Source: CAD feature listing. Evaluate the final solid. Frame: model axes, mm. Face numbers are marked on the shaded views. Give positions to 0.01 mm unless a question says otherwise; leave off trailing zeros. Order: outer loops, then holes, each group sorted by start corner. A loop starts at its lowest first (then second) coordinate and runs counter-clockwise, first axis right, second up. Notation, with made-up numbers: (45, 33) -> (78, 33) arc R16 cw to (78, 61) -> close; hole circle Ø8 at (36.25, 8). An arc over 180 degrees is marked (long way). Answer in a Markdown table with one row per item.
```python
from build123d import *

# Parameters (mm, degrees)
F0_R     = 11
F1_DEPTH = 7


with BuildPart() as f1:
    # F0 (on Top) → F1 (new body)
    with BuildSketch(Plane.XY):
        with BuildLine():
            ThreePointArc((14.1759402298, -3.0483960701), (14.4187574592, -1.5327861344), (14.5, 0))
            ThreePointArc((14.5, 0), (14.421984404, 1.5021204517), (14.188777124, 2.9880769278))
            add(Edge.make_bspline(
                [(14.0117061641, 3.7312317498), (14.0561894605, 3.4787953407), (14.1150221965, 3.2304441785), (14.188777124, 2.9880769278)],
                knots=[0.9498383363, 0.9498383363, 0.9498383363, 0.9498383363, 1, 1, 1, 1], degree=3))
            ThreePointArc((14.0117061641, 3.7312317498), (7.1105429941, 12.6368579295), (-4.0835358776, 13.9131137685))
            add(Edge.make_bspline(
                [(-4.0835358776, 13.9131137685), (-4.9864056262, 13.4237848609), (-5.8861011392, 13.0613615019), (-6.6725668518, 12.8734941492)],
                knots=[0.8398981571, 0.8398981571, 0.8398981571, 0.8398981571, 1, 1, 1, 1], degree=3))
            ThreePointArc((-6.6725668518, 12.8734941492), (-7.25, 12.5573683549), (-7.8124895427, 12.2153594767))
            add(Edge.make_bspline(
                [(-10.3373118209, 10.1680865613), (-9.3752684105, 10.9198780403), (-8.503153556, 11.689001034), (-7.8124895427, 12.2153594767)],
                knots=[0.8153153807, 0.8153153807, 0.8153153807, 0.8153153807, 1, 1, 1, 1], degree=3))
            ThreePointArc((-10.3373118209, 10.1680865613), (-14.5, 0), (-10.3373118209, -10.1680865613))
            add(Edge.make_bspline(
                [(-10.3373118209, -10.1680865613), (-9.3752684105, -10.9198780403), (-8.503153556, -11.689001034), (-7.8124895427, -12.2153594767)],
                knots=[0.8153153807, 0.8153153807, 0.8153153807, 0.8153153807, 1, 1, 1, 1], degree=3))
            ThreePointArc((-7.8124895427, -12.2153594767), (-6.1812855522, -13.1164670899), (-4.4479816774, -13.8009223966))
            add(Edge.make_bspline(
                [(-3.7286645674, -14.0123895373), (-3.9647890084, -13.9271776533), (-4.2049522049, -13.8562123362), (-4.4479816774, -13.8009223966)],
                knots=[0.9507919436, 0.9507919436, 0.9507919436, 0.9507919436, 1, 1, 1, 1], degree=3))
            ThreePointArc((-3.7286645674, -14.0123895373), (7.25, -12.5573683549), (13.9994175907, -3.7770765311))
            add(Edge.make_bspline(
                [(13.9994175907, -3.7770765311), (14.043684155, -3.5299808247), (14.1023079859, -3.2865107369), (14.1759402298, -3.0483960701)],
                knots=[0.9507919436, 0.9507919436, 0.9507919436, 0.9507919436, 1, 1, 1, 1], degree=3))
        make_face()
        Circle(F0_R, mode=Mode.SUBTRACT)
        with BuildLine():
            ThreePointArc((-4.0835358776, 13.9131137685), (7.1105429941, 12.6368579295), (14.0117061641, 3.7312317498))
            add(Edge.make_bspline(
                [(16.8041360144, 10.9260038108), (16.4779875659, 10.7042997166), (14.5192375285, 9.1026767142), (13.6103052967, 6.0091248438), (14.0117061641, 3.7312317498)],
                knots=[0.4134483725, 0.4134483725, 0.4134483725, 0.4134483725, 0.4971979755, 0.9498383363, 0.9498383363, 0.9498383363, 0.9498383363], degree=3))
            ThreePointArc((16.8041360144, 10.9260038108), (7.4408037917, 12.6342244362), (1.1538261794, 19.7801267949))
            add(Edge.make_bspline(
                [(1.1538261794, 19.7801267949), (1.1027747103, 19.4661195397), (0.518142053, 17.2084365704), (-1.9632609294, 15.0622405677), (-4.0835358776, 13.9131137685)],
                knots=[0.4034852163, 0.4034852163, 0.4034852163, 0.4034852163, 0.4639193106, 0.8398981571, 0.8398981571, 0.8398981571, 0.8398981571], degree=3))
        make_face()
        with BuildLine():
            add(Edge.make_bspline(
                [(16.8324180589, -10.9304210804), (16.5090270331, -10.7103658028), (14.5525951809, -9.1161932679), (13.5913899182, -6.0546846446), (13.9994175907, -3.7770765311)],
                knots=[0.4137406454, 0.4137406454, 0.4137406454, 0.4137406454, 0.4972159985, 0.9507919436, 0.9507919436, 0.9507919436, 0.9507919436], degree=3))
            ThreePointArc((13.9994175907, -3.7770765311), (7.25, -12.5573683549), (-3.7286645674, -14.0123895373))
            add(Edge.make_bspline(
                [(1.0498133002, -20.0425121863), (1.0209353525, -19.6524197039), (0.6185573654, -17.1610137516), (-1.552184245, -14.7978312642), (-3.7286645674, -14.0123895373)],
                knots=[0.4137406454, 0.4137406454, 0.4137406454, 0.4137406454, 0.4972159985, 0.9507919436, 0.9507919436, 0.9507919436, 0.9507919436], degree=3))
            ThreePointArc((1.0498133002, -20.0425121863), (7.3307033346, -12.6971506308), (16.8324180589, -10.9304210804))
        make_face()
        with BuildLine():
            ThreePointArc((1.1538261794, 19.7801267949), (7.4408037917, 12.6342244362), (16.8041360144, 10.9260038108))
            add(Edge.make_bspline(
                [(22.4852798786, 13.0985463935), (20.5195105726, 12.423663188), (18.4142397082, 12.0204949315), (16.8041360144, 10.9260038108)],
                knots=[0, 0, 0, 0, 0.4134483725, 0.4134483725, 0.4134483725, 0.4134483725], degree=3))
            ThreePointArc((22.4852798786, 13.0985463935), (27.3256309509, 18.3395482658), (29.0807033346, 25.2545189857))
            ThreePointArc((29.0807033346, 25.2545189857), (14.964626833, 39.7494354307), (0.1010339902, 26.0220967828))
            add(Edge.make_bspline(
                [(0.1010339902, 26.0220967828), (0.5023641828, 24.0338894608), (1.4946687664, 21.8765805705), (1.1538261794, 19.7801267949)],
                knots=[0, 0, 0, 0, 0.4034852163, 0.4034852163, 0.4034852163, 0.4034852163], degree=3))
        make_face()
        with Locations((14.5807033346, 25.2545189857)):
            Circle(F0_R, mode=Mode.SUBTRACT)
        with BuildLine():
            add(Edge.make_bspline(
                [(22.4852798786, -13.0985463935), (20.5122225081, -12.4305468552), (18.4352865313, -12.0211120353), (16.8324180589, -10.9304210804)],
                knots=[0, 0, 0, 0, 0.4137406454, 0.4137406454, 0.4137406454, 0.4137406454], degree=3))
            ThreePointArc((16.8324180589, -10.9304210804), (7.3307033346, -12.6971506308), (1.0498133002, -20.0425121863))
            add(Edge.make_bspline(
                [(0.1010339902, -26.0220967828), (0.5090581055, -23.9793792077), (1.1929451387, -21.9759824798), (1.0498133002, -20.0425121863)],
                knots=[0, 0, 0, 0, 0.4137406454, 0.4137406454, 0.4137406454, 0.4137406454], degree=3))
            ThreePointArc((0.1010339902, -26.0220967828), (14.964626833, -39.7494354307), (29.0807033346, -25.2545189857))
            ThreePointArc((29.0807033346, -25.2545189857), (27.3256309509, -18.3395482658), (22.4852798786, -13.0985463935))
        make_face()
        with Locations((14.5807033346, -25.2545189857)):
            Circle(F0_R, mode=Mode.SUBTRACT)
        with BuildLine():
            ThreePointArc((-10.3373118209, -10.1680865613), (-14.5, 0), (-10.3373118209, 10.1680865613))
            add(Edge.make_bspline(
                [(-17.2748335615, 8.3041784514), (-16.7684606801, 8.0190428188), (-14.5727828059, 7.2074422158), (-12.0132482268, 8.8584214299), (-10.3373118209, 10.1680865613)],
                knots=[0.3927670048, 0.3927670048, 0.3927670048, 0.3927670048, 0.4935838728, 0.8153153807, 0.8153153807, 0.8153153807, 0.8153153807], degree=3))
            ThreePointArc((-17.2748335615, 8.3041784514), (-15.3301863677, 4.3528548067), (-14.6614066693, 0))
            ThreePointArc((-14.6614066693, 0), (-15.3301863677, -4.3528548067), (-17.2748335615, -8.3041784514))
            add(Edge.make_bspline(
                [(-17.2748335615, -8.3041784514), (-16.7684606801, -8.0190428188), (-14.5727828059, -7.2074422158), (-12.0132482268, -8.8584214299), (-10.3373118209, -10.1680865613)],
                knots=[0.3927670048, 0.3927670048, 0.3927670048, 0.3927670048, 0.4935838728, 0.8153153807, 0.8153153807, 0.8153153807, 0.8153153807], degree=3))
        make_face()
        with BuildLine():
            ThreePointArc((-14.6614066693, 0), (-15.3301863677, 4.3528548067), (-17.2748335615, 8.3041784514))
            add(Edge.make_bspline(
                [(-22.5863138688, 12.9235503893), (-20.9547365723, 11.9145258046), (-19.2475843898, 9.4150230013), (-17.2748335615, 8.3041784514)],
                knots=[0, 0, 0, 0, 0.3927670048, 0.3927670048, 0.3927670048, 0.3927670048], degree=3))
            ThreePointArc((-22.5863138688, 12.9235503893), (-43.6614066693, 0), (-22.5863138688, -12.9235503893))
            add(Edge.make_bspline(
                [(-22.5863138688, -12.9235503893), (-20.9547365723, -11.9145258046), (-19.2475843898, -9.4150230013), (-17.2748335615, -8.3041784514)],
                knots=[0, 0, 0, 0, 0.3927670048, 0.3927670048, 0.3927670048, 0.3927670048], degree=3))
            ThreePointArc((-17.2748335615, -8.3041784514), (-15.3301863677, -4.3528548067), (-14.6614066693, 0))
        make_face()
        with Locations((-29.1614066693, 0)):
            Circle(F0_R, mode=Mode.SUBTRACT)
    extrude(amount=F1_DEPTH)


solid = f1.part
```
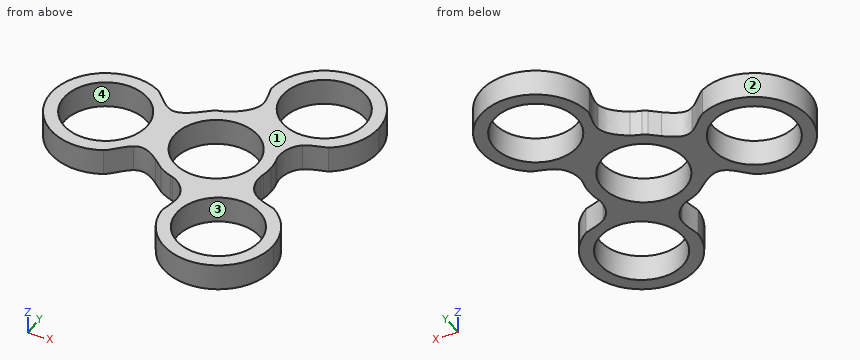
(1) First-contact query: pin 1 Ø12 at (x, y) = (-5, -29.5) entering from +Z; pin 2 Ø3 at (x, z) = (-10, 5) entering from +Y; pin 3 Ø2 at (x, z) = (-18.5, 5) entering from -Y. Flat tips, straight axial feed; report the tip coordinate or a pass-through.
A:
| item | result |
|---|---|
| pin 1 | stops at z = 7 |
| pin 2 | stops at y = 11.67 |
| pin 3 | stops at y = -10.09 |
(2) Section query A-A (y = -29). Return the cut outline in (x, z).
A:
| item | result |
|---|---|
| outline | (0.57, 0) -> (4.24, 0) -> (4.24, 7) -> (0.57, 7) -> close; (24.92, 0) -> (28.59, 0) -> (28.59, 7) -> (24.92, 7) -> close |
(3) Section query C-C (x = -26). Return the cut outline in (y, z), plus the area to 3 significant figures.
A:
| item | result |
|---|---|
| outline | (-14.15, 0) -> (-10.54, 0) -> (-10.54, 7) -> (-14.15, 7) -> close; (10.54, 0) -> (14.15, 0) -> (14.15, 7) -> (10.54, 7) -> close |
| area | 50.6 mm^2 |
(4) Ray query, probe 1 along X at (y, z) = (-7, 1.25); probe 2 along X at (y, z) = (-3.5, 3); probe 3 along Y at (x, z) = (9.5, 0.5). Return the intervals inside material, ascending.
A:
| item | result |
|---|---|
| probe 1 | x = -41.86 to -37.65, -20.68 to -8.49, 8.49 to 14.17 |
| probe 2 | x = -43.23 to -39.59, -18.73 to -10.43, 10.43 to 14.06 |
| probe 3 | y = -38.84 to -35.01, -15.5 to -5.55, 5.55 to 15.5, 35.01 to 38.84 |
(5) Section query B-B (x = 6.5). Return the cut outline in (y, z), plus the area to 3 significant figures.
A:
| item | result |
|---|---|
| outline | (-37.29, 0) -> (-32.72, 0) -> (-32.72, 7) -> (-37.29, 7) -> close; (-17.79, 0) -> (-8.87, 0) -> (-8.87, 7) -> (-17.79, 7) -> close; (8.87, 0) -> (17.79, 0) -> (17.79, 7) -> (8.87, 7) -> close; (32.72, 0) -> (37.29, 0) -> (37.29, 7) -> (32.72, 7) -> close |
| area | 189 mm^2 |
(6) Pull-direction query (Y, two-part tool) for the marked faces 1, 2, 3 and 4; classes: +Y half, -Y half, draft (parallel to the pull), parting line (faces both ways), or undercut.
A:
| item | result |
|---|---|
| face 1 | draft |
| face 2 | parting line |
| face 3 | undercut |
| face 4 | undercut |
(7) Section query D-D (y = -6). Give the number of separate pieces and of enclosed holes in the cut face, plus the area to 3 significant figures.
A:
| item | result |
|---|---|
| separate pieces | 3 |
| enclosed holes | 0 |
| area | 136 mm^2 |
